For this review, take the finished solid that the model builds, in its own axes (mm). A direction names the side the tool comes from. Coordinates: 2 decimals unless noted, no trailing zeros. Write each loop counter-clockwise with the first axis right and the second up, starting at its lowest first coordinate (ties: lowest second). Pieces come first, ordered by that corner, then holes.
```python
from build123d import *

# Parameters (mm, degrees)
CROQUIS1_W            = 50.8
CROQUIS1_H            = 6.31
CROQUIS2_R            = 6.35
CORTAR_EXTRUIR1_DEPTH = 6.31


with BuildPart() as part:
    # Barrer1: sweep along a curve in space
    with BuildLine() as barrer1_path:
        Line((0, 0, 0), (0, 0, 958.84))
        Line((0, 0, 958.84), (0, -64.9, 958.84))
        Line((0, -64.9, 958.84), (90, -64.9, 958.84))
    # Croquis1 → Barrer1 (sweep)
    with BuildSketch(Plane.XY):
        Rectangle(CROQUIS1_W, CROQUIS1_H)
    sweep(path=barrer1_path.line, transition=Transition.RIGHT)

    # Croquis2 → Cortar-Extruir1 (cut)
    with BuildSketch(Plane(origin=(0, 3.155, 0), x_dir=(1, 0, 0), z_dir=(0, 1, 0))):
        with Locations(Location((0, -43.892204666, 0), (0, 0, 270))):
            Circle(CROQUIS2_R)
        with Locations(Location((0, -11.892204666, 0), (0, 0, 270))):
            Circle(CROQUIS2_R)
    extrude(amount=-CORTAR_EXTRUIR1_DEPTH, mode=Mode.SUBTRACT)


solid = part.part
```
Q1. Clearance check with flat-ended pins moving along their axes: pin 1 Ø8 at (x, y) = (38.5, -38.5) entering from +Z (3 decimals); pin 2 Ø3 at (x, y) = (38.5, -80) entering from -Z (3 decimals); pin 3 Ø16.5 at (x, z) = (0, 11.89) entering from -Y (3 decimals); pin 4 Ø1.9 at (x, z) = (70, 958) entering from +Y. State where each tip first meets the part, or that it passes through.
Ans:
pin 1: stops at z = 961.995
pin 2: stops at z = 955.685
pin 3: stops at y = -3.155
pin 4: stops at y = -39.5
Q2. Add section B-B (x = 60). State the section outline as (y, z) points (3 decimals).
Ans:
outline: (-90.3, 955.685) - (-39.5, 955.685) - (-39.5, 961.995) - (-90.3, 961.995) - close
Q3. Tool access review of faces 1 (the flat face through (19, -57, 955.685)), 2 (the flat face through (0, 3.155, 488)): name each direction out of +Z, -Z, +X, -X, +Y, -Y from which nothing blocks a thin tool from reaching the whole face with its end or side.
Ans:
face 1: -Z, +X, -X, -Y
face 2: +Z, -Z, +X, -X, +Y
Q4. Add section A-A (z = 892.5). State the section outline as (x, y) points (3 decimals), then the cut area to 3 significant figures.
Ans:
outline: (-25.4, -3.155) - (25.4, -3.155) - (25.4, 3.155) - (-25.4, 3.155) - close
area: 321 mm2
Q5. For probe 1 along Z at (x, y) = (62.5, -82.5) (3 decimals); probe 2 along Y at (x, z) = (23.5, 638) (3 decimals), list the stretches that pass through material, from the lowest coordinate up.
Ans:
probe 1: z = 955.685 to 961.995
probe 2: y = -3.155 to 3.155
